from build123d import *

# Parameters (mm, degrees)
F0_R     = 6.35
F0_R_2   = 3.175
F1_DEPTH = 3.175


with BuildPart() as f1:
    # F0 (on Top) → F1 (new body)
    with BuildSketch(Plane.XY):
        with BuildLine():
            Line((-50.8, 222.153178), (-50.8, 0))
            Line((-50.8, 0), (-50.8, -222.153178))
            ThreePointArc((-50.8, -222.153178), (-50.601455, -223.258321), (-50.030652, -224.225246))
            Line((-50.030652, -224.225246), (-27.137392, -250.804108))
            ThreePointArc((-27.137392, -250.804108), (-26.054958, -251.618165), (-24.731741, -251.90704))
            Line((-24.731741, -251.90704), (24.731741, -251.90704))
            ThreePointArc((24.731741, -251.90704), (26.054958, -251.618165), (27.137392, -250.804108))
            Line((27.137392, -250.804108), (50.030652, -224.225246))
            ThreePointArc((50.030652, -224.225246), (50.601455, -223.258321), (50.8, -222.153178))
            Line((50.8, -222.153178), (50.8, 0))
            Line((50.8, 0), (50.8, 222.153178))
            ThreePointArc((50.8, 222.153178), (50.601455, 223.258321), (50.030652, 224.225246))
            Line((50.030652, 224.225246), (27.137392, 250.804108))
            ThreePointArc((27.137392, 250.804108), (26.054958, 251.618165), (24.731741, 251.90704))
            Line((24.731741, 251.90704), (-24.731741, 251.90704))
            ThreePointArc((-24.731741, 251.90704), (-26.054958, 251.618165), (-27.137392, 250.804108))
            Line((-27.137392, 250.804108), (-50.030652, 224.225246))
            ThreePointArc((-50.030652, 224.225246), (-50.601455, 223.258321), (-50.8, 222.153178))
        make_face()
        with Locations((0, -223.33204)):
            Circle(F0_R, mode=Mode.SUBTRACT)
        with Locations((-25.4, -50.8)):
            Circle(F0_R_2, mode=Mode.SUBTRACT)
        with Locations((25.4, -50.8)):
            Circle(F0_R_2, mode=Mode.SUBTRACT)
        with Locations((-25.4, 50.8)):
            Circle(F0_R_2, mode=Mode.SUBTRACT)
        with Locations((0, 223.33204)):
            Circle(F0_R, mode=Mode.SUBTRACT)
        with Locations((25.4, 50.8)):
            Circle(F0_R_2, mode=Mode.SUBTRACT)
    extrude(amount=F1_DEPTH)


solid = f1.part
Geometry check sheet. Reference: the model listing, model coordinates, mm. Coordinates: 2 decimals unless noted, no trailing zeros. Order: outer loops, then holes, each group sorted by start corner. A loop starts at its lowest first (then second) coordinate and runs counter-clockwise, first axis right, second up. Notation, with made-up numbers: (41, -11) -> (64, -11) arc R30 ccw to (64, 12) -> close; hole circle Ø7 at (87.5, 28). An arc over 180 degrees is marked (long way). Use a Markdown table: item, result. Add a question column.
1. Cross-section at A-A (x = 0). Enter the section's corners in (y, z) (3 decimals), and give its area (3 significant figures).
2. Cross-section at B-B (z = 0.7). Enter the section's corners in (x, y) (3 decimals).
3. Go/stop test with flat-tipped pins: pin 1 Ø5 at (x, y) = (-25.4, 50.8) entering from -Z; pin 2 Ø1 at (x, z) = (28.5, 1) entering from -Y; pin 3 Ø1 at (x, z) = (-33, 1.5) entering from -Y. Record where each tip stops, or that it passes through.
4. Cross-section at C-C (x = -38.5). Enter the section's corners in (y, z) (3 decimals).
5. Material ranges on L1, parallel to Y at x = 25.4, z = 1.1 (3 decimals); L2, parallel to Y at x = 0, z = 2.1; L3, parallel to Y at x = 38, z = 0.35, recorded low to high.
6. Cross-section at D-D (x = 41). Enter the section's corners in (y, z) (3 decimals), and give its area (3 significant figures).
7. Mould release check, pull along X, two halves, no side actions. Record for faces 1 (the face through (-38.744, -237.329, 1.565)), 2 (the face through (-1.377, 217.133, 1.565)), 3 (the face through (38.744, 237.329, 1.565)), 4 (the face through (-4.68, -219.04, 1.57)): pulls with the +X half, pulls with the -X half, needs draft (parallel to the pull), parting line crosses it, or undercut.
Filled sheet:
| question | item | result |
|---|---|---|
| 1 | outline | (-251.907, 0) -> (-229.682, 0) -> (-229.682, 3.175) -> (-251.907, 3.175) -> close; (-216.982, 0) -> (216.982, 0) -> (216.982, 3.175) -> (-216.982, 3.175) -> close; (229.682, 0) -> (251.907, 0) -> (251.907, 3.175) -> (229.682, 3.175) -> close |
| 1 | area | 1,520 mm2 |
| 2 | outline | (-50.8, -222.153) arc R3.175 ccw to (-50.031, -224.225) -> (-27.137, -250.804) arc R3.175 ccw to (-24.732, -251.907) -> (24.732, -251.907) arc R3.175 ccw to (27.137, -250.804) -> (50.031, -224.225) arc R3.175 ccw to (50.8, -222.153) -> (50.8, 222.153) arc R3.175 ccw to (50.031, 224.225) -> (27.137, 250.804) arc R3.175 ccw to (24.732, 251.907) -> (-24.732, 251.907) arc R3.175 ccw to (-27.137, 250.804) -> (-50.031, 224.225) arc R3.175 ccw to (-50.8, 222.153) -> close; hole circle Ø6.35 at (-25.4, -50.8); hole circle Ø6.35 at (-25.4, 50.8); hole circle Ø12.7 at (0, -223.332); hole circle Ø12.7 at (0, 223.332); hole circle Ø6.35 at (25.4, -50.8); hole circle Ø6.35 at (25.4, 50.8) |
| 3 | pin 1 | through |
| 3 | pin 2 | y = -249.8 |
| 3 | pin 3 | y = -244.58 |
| 4 | outline | (-237.612, 0) -> (237.612, 0) -> (237.612, 3.175) -> (-237.612, 3.175) -> close |
| 5 | L1 | -251.836 to -53.975, -47.625 to 47.625, 53.975 to 251.836 |
| 5 | L2 | -251.91 to -229.68, -216.98 to 216.98, 229.68 to 251.91 |
| 5 | L3 | -238.19 to 238.19 |
| 6 | outline | (-234.71, 0) -> (234.71, 0) -> (234.71, 3.175) -> (-234.71, 3.175) -> close |
| 6 | area | 1,490 mm2 |
| 7 | face 1 | pulls with the -X half |
| 7 | face 2 | undercut |
| 7 | face 3 | pulls with the +X half |
| 7 | face 4 | undercut |
